Source: CAD feature listing. Evaluate the final solid. Frame: model axes, mm. Round coordinates to 2 decimals unless told otherwise and drop trailing zeros. Order: outer loops, then holes, each group sorted by start corner. A loop starts at its lowest first (then second) coordinate and runs counter-clockwise, first axis right, second up. Notation, with made-up numbers: M -27.5,64.5 L -20.5,64.5 A30 ccw -20.5,97.5 Z; hole C 79.25,-16 d7. An arc over 180 degrees is marked long. Use one line per item in the form item = value. Start each with the question number.
Q1. Contact query for flat-ended pins moving along their axis: pin 1 (3 mm diameter, centred on x = 126, y = 200, fed in from -Z); pin 2 (5 mm diameter, centred on x = 125, z = -35.5, fed in from -Y); pin 3 (8 mm diameter, centred on x = 125, y = 180.5, fed in from +Z). Output: stop coordinate, or through.
Q2. Section D-D (x = -77). Return the cut outline in (y, z), plus the area to 3 significant figures.
Q3. Section C-C (y = 206). Return the cut outline in (x, z).
Q4. Material intervals for probe 1 along Z at (x, y) = (-40, 5); probe 2 along Y at (x, z) = (-85.5, -74); probe 3 along Z at (x, y) = (-73.5, 454.5), sorted ascending.
Q5. Section A-A (x = -40.68). Return the cut outline in (y, z).
Q6. Section B-B (z = 166). Return the cut outline in (x, y).
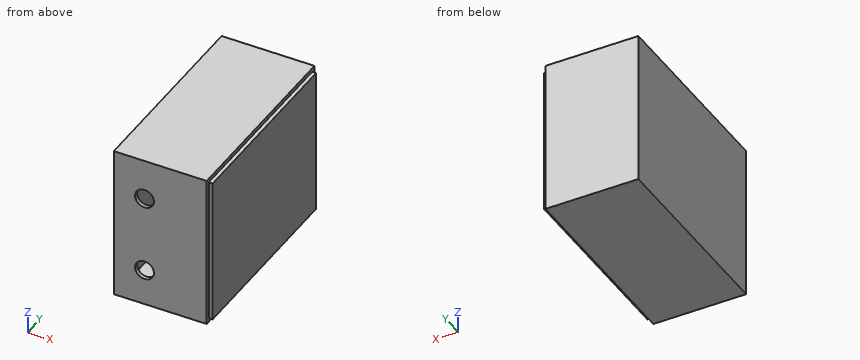
Autodesk Inventor part; units mm, degrees
ref_plane "YZ Plane" through (0, 0, 0) normal (1, 0, 0) x (0, 1, 0)
ref_plane "XZ Plane" through (0, 0, 0) normal (0, 1, 0) x (-1, 0, 0)
ref_plane "XY Plane" through (0, 0, 0) normal (0, 0, 1) x (1, 0, 0)
sketch "Sketch1" plane through (0, 0, 0) normal (0, 1, 0) x (-1, 0, 0)
  line L0 (-120, 200) -> (120, 200)
  line L1 (120, 200) -> (120, -200)
  line L2 (120, -200) -> (-120, -200)
  line L3 (-120, -200) -> (-120, 200)
  line L4 (-120, 200) -> (120, -200) construction
  line L5 (120, 200) -> (-120, -200) construction
  point P0 (0, 0)
  dimension "d0" = 400
  dimension "d1" = 240
extrude "Extrusion1" add sketch "Sketch1" along normal blind 508
sketch "Sketch2" plane through (0, 0, 0) normal (0, -1, 0) x (1, 0, 0)
  point P0 (0, 0)
sketch "Sketch3" plane through (0, 0, 0) normal (0, -1, 0) x (1, 0, 0)
  circle A0 centre (-40.68, 94.7135) radius 24.5
  circle A1 centre (-40.68, -105.2865) radius 24.5
  line L0 (-120, 200) -> (-120, -200)
  point P0 (0, 0)
  dimension "d4" = 49
  dimension "d5" = 49
  dimension "d6" = 200
  dimension "d17" = 79.32
  dimension "d18" = 79.32
shell "Shell1" thickness 10 removed faces 0
extrude "Extrusion2" cut sketch "Sketch3" against normal blind 10
sketch "Sketch4" plane through (120, 0, 200) normal (1, 0, 0) x (0, 0, -1)
  line L0 (10, 498) -> (390, 498)
  line L1 (390, 10) -> (390, 498)
  line L2 (10, 498) -> (390, 498)
  line L3 (390, 498) -> (390, 10)
  line L4 (390, 10) -> (10, 10)
  line L5 (10, 10) -> (10, 498)
  point P0 (200, 0)
extrude "Extrusion3" add sketch "Sketch4" along normal blind 10
properties part number "powerBox"
Results list:
q1.pin_1 = -190
q1.pin_2 = 10
q1.pin_3 = 190
q2.outline = M 0,-200 L 508,-200 L 508,200 L 0,200 Z; hole M 10,-190 L 498,-190 L 498,190 L 10,190 Z
q2.area = 17,800 mm2
q3.outline = M -120,-200 L 120,-200 L 120,-190 L 130,-190 L 130,190 L 120,190 L 120,200 L -120,200 Z; hole M -110,-190 L 110,-190 L 110,190 L -110,190 Z
q4.probe_1 = -200 to -129.78, -80.8 to 70.22, 119.2 to 200
q4.probe_2 = 0 to 10, 498 to 508
q4.probe_3 = -200 to -190, 190 to 200
q5.outline = M 0,-200 L 508,-200 L 508,200 L 0,200 L 0,119.21 L 10,119.21 L 10,190 L 498,190 L 498,-190 L 10,-190 L 10,-129.79 L 0,-129.79 Z; M 0,-80.79 L 10,-80.79 L 10,70.21 L 0,70.21 Z
q6.outline = M -120,0 L 120,0 L 120,10 L 130,10 L 130,498 L 120,498 L 120,508 L -120,508 Z; hole M -110,10 L 110,10 L 110,498 L -110,498 Z
